Geometry: final body of the model. Coordinates: model frame, mm. A direction names the side the tool comes from. Coordinates: 2 decimals unless noted, no trailing zeros. Write each loop counter-clockwise with the first axis right and the second up, starting at its lowest first coordinate (ties: lowest second). Pieces come first, ordered by that corner, then holes. Notation, with made-up numbers: M -16,41 L 30,41 A13 ccw 30,56 Z; hole C -22.5,15.25 d9. An arc over 180 degrees is marked long. Write item = value, one per line. Start each with the question number.
Item 1: Reachability of faces 1 (the cylindrical face through (0.207, -4.74, -16.485)), 2 (the cylindrical face through (-21.199, 6.261, 6.676)), 3 (the cylindrical face through (-5.506, -3.153, -24.796)) from +Z, -Z, +X, -X, +Y, -Y: full face, straight path, thin tool, end or side. Return the list, or none.
Item 2: Section A-A on y = 12. Output: boundary loops of the cut face in (x, z) (3 decimals), plus the area to 3 significant figures.
Item 3: Pull-direction query (Z, two-part tool) for faces 4 (the conical face through (0.148, -2.387, -17.827)), 5 (the conical face through (17.78, -2.39, 0.01)), 6 (the flat face through (-20, 0, 11)), 7 (the cylindrical face through (5.506, 15.853, -24.796)); classes: +Z half, -Z half, draft (parallel to the pull), parting line (faces both ways), or undercut.
Item 4: First-contact query: pin 1 Ø3 at (y, z) = (15.5, 2.5) entering from -X; pin 2 Ø1.5 at (y, z) = (10, 10) entering from +X; pin 3 Ø5 at (y, z) = (0.5, -15) entering from -X. Flat tips, straight axial feed; report the tip coordinate or a pass-through.
Item 5: Ray query, L1, parallel to Z at x = 0, y = 0.75 (3 decimals); L2, parallel to Y at x = 21, z = 8; L3, parallel to X at y = -0.5, z = 1. Return the intervals inside material, ascending. Write a range as [from, to].
from build123d import *

# Parameters (mm, degrees)
F0_R     = 25.4
F1_DEPTH = 6.35
F2_R     = 22.225
F3_DEPTH = 12.7
F4_R     = 25.4
F5_DEPTH = 6.35
F6_R     = 1.6002
F8_D     = 3.175
F8_DEPTH = 3.175
F8_TIP   = 0.9538662327
F10_D    = 12.7


with BuildPart() as f1:
    # F0 (on Front) → F1 (new body)
    with BuildSketch(Plane.XZ):
        Circle(F0_R)
    extrude(amount=F1_DEPTH)

    # F2 (on face) → F3 (join)
    with BuildSketch(Plane(origin=(0, 0, 0), x_dir=(-1, 0, 0), z_dir=(0, 1, 0))):
        Circle(F2_R)
    extrude(amount=F3_DEPTH)

    # F4 (on face) → F5 (join)
    with BuildSketch(Plane(origin=(0, 12.7, 0), x_dir=(-1, 0, 0), z_dir=(0, 1, 0))):
        Circle(F4_R)
    extrude(amount=F5_DEPTH)

    # F6
    f6_edges = [f1.edges().sort_by_distance(p)[0] for p in [
        (-25.4, -6.35, 0),
        (25.4, 19.05, 0),
        (-25.4, 0, 0),
        (25.4, 12.7, 0),
    ]]
    fillet(f6_edges, radius=F6_R)

    # F8
    with Locations(Plane.XZ.offset(6.35)):
        with Locations((0, 18.0589817464), (-18.0589817464, 0), (0, -18.0589817464), (18.0589817464, 0)):
            Hole(F8_D / 2, depth=F8_DEPTH)
            with Locations((0, 0, -(F8_DEPTH + F8_TIP / 2))):  # 118° drill point
                Cone(0, F8_D / 2, F8_TIP, mode=Mode.SUBTRACT)

    # F10 (through all)
    with Locations(Plane.XZ.offset(6.35)):
        with Locations((0, 0)):
            Hole(F10_D / 2)


solid = f1.part
Responses:
q1.face_1 = -Y
q1.face_2 = none
q1.face_3 = +Y, -Y
q2.outline = C 0,0 d44.45; hole C 0,0 d12.7
q2.area = 1,430 mm²
q3.face_4 = undercut
q3.face_5 = undercut
q3.face_6 = draft
q3.face_7 = parting line
q4.pin_1 = -25.38
q4.pin_2 = 20.21
q4.pin_3 = -21.69
q5.L1 = [-22.225, -6.35], [6.35, 22.225]
q5.L2 = [-6.35, 0], [12.7, 19.05]
q5.L3 = [-24.94, -6.27], [6.27, 24.94]
